Could you check a few things on this model? Use its own coordinates, in mm. Give positions to 0.01 mm unless a question says otherwise; leave off trailing zeros. Order: outer loops, then holes, each group sorted by start corner. A loop starts at its lowest first (then second) coordinate and runs counter-clockwise, first axis right, second up. Notation, with made-up numbers: M 35,13 L 65,13 A14 ccw 65,34 Z; hole C -1,86.5 d5. An arc over 180 degrees is marked long. Return JSON: item names as keys, results as strings. Group by question number.
```python
from build123d import *

# Parameters (mm, degrees)
F1_DEPTH = 5.08


# Not quite as in the source:
# - a feature names something its author has since deleted; it is built from what else it names


with BuildPart() as f1:
    # F0 (on Top) → F1 (new body)
    with BuildSketch(Plane.XY):
        with BuildLine():
            ThreePointArc((7.5830097901, 0.7499083436), (7.6107468293, 0.3754100423), (7.62, 0))
            ThreePointArc((7.62, 0), (0.4990141385, -7.6036428697), (-7.5546417033, -0.9958859045))
            ThreePointArc((-7.5546417033, -0.9958859045), (-6.3173271202, -6.8123022238), (-3.6964522326, -12.1501539452))
            ThreePointArc((-3.6964522326, -12.1501539452), (7.5612517696, -10.2037969245), (12.7, 0))
            ThreePointArc((12.7, 0), (12.5868786701, 1.6912969415), (12.249529867, 3.3524644721))
            ThreePointArc((12.249529867, 3.3524644721), (9.1791212991, 8.776886246), (3.897633179, 12.0871194088))
            ThreePointArc((3.897633179, 12.0871194088), (6.451051693, 6.6495502812), (7.5830097901, 0.7499083436))
        make_face()
        with BuildLine():
            ThreePointArc((-36.917633179, 12.0871194088), (-16.51, 23.3293611901), (3.897633179, 12.0871194088))
            ThreePointArc((3.897633179, 12.0871194088), (9.1791212991, 8.776886246), (12.249529867, 3.3524644721))
            ThreePointArc((12.249529867, 3.3524644721), (-18.3173290135, 29.0331939814), (-45.72, 0))
            ThreePointArc((-45.72, 0), (-43.286205272, 7.4762978347), (-36.917633179, 12.0871194088))
        make_face()
        with BuildLine():
            ThreePointArc((-20.32, 0), (-25.5437021653, 10.266205272), (-36.917633179, 12.0871194088))
            ThreePointArc((-36.917633179, 12.0871194088), (-43.286205272, 7.4762978347), (-45.72, 0))
            ThreePointArc((-45.72, 0), (-33.02, -12.7), (-20.32, 0))
        make_face()
        with BuildLine():
            ThreePointArc((-40.64, 0), (-40.6307468293, 0.3754100423), (-40.6030097901, 0.7499083436))
            ThreePointArc((-40.6030097901, 0.7499083436), (-32.6445899577, 7.6107468293), (-25.4, 0))
            ThreePointArc((-25.4, 0), (-33.02, -7.62), (-40.64, 0))
        make_face(mode=Mode.SUBTRACT)
        with BuildLine():
            ThreePointArc((36.7164522326, -12.1501539452), (16.51, -23.0707915841), (-3.6964522326, -12.1501539452))
            ThreePointArc((-3.6964522326, -12.1501539452), (-9.1059552655, -8.8527723739), (-12.249529867, -3.3524644721))
            ThreePointArc((-12.249529867, -3.3524644721), (18.3173290135, -29.0331939814), (45.72, 0))
            ThreePointArc((45.72, 0), (43.2237969245, -7.5612517696), (36.7164522326, -12.1501539452))
        make_face()
        with BuildLine():
            ThreePointArc((45.72, 0), (22.8162030755, 7.5612517696), (36.7164522326, -12.1501539452))
            ThreePointArc((36.7164522326, -12.1501539452), (43.2237969245, -7.5612517696), (45.72, 0))
        make_face()
        with BuildLine():
            ThreePointArc((40.64, 0), (40.6236428697, -0.4990141385), (40.5746417033, -0.9958859045))
            ThreePointArc((40.5746417033, -0.9958859045), (25.4163571303, 0.4990141385), (40.64, 0))
        make_face(mode=Mode.SUBTRACT)
        with BuildLine():
            ThreePointArc((-7.62, 0), (-0.3754100423, 7.6107468293), (7.5830097901, 0.7499083436))
            ThreePointArc((7.5830097901, 0.7499083436), (6.451051693, 6.6495502812), (3.897633179, 12.0871194088))
            ThreePointArc((3.897633179, 12.0871194088), (-8.776886246, 9.1791212991), (-12.249529867, -3.3524644721))
            ThreePointArc((-12.249529867, -3.3524644721), (-9.1059552655, -8.8527723739), (-3.6964522326, -12.1501539452))
            ThreePointArc((-3.6964522326, -12.1501539452), (-6.3173271202, -6.8123022238), (-7.5546417033, -0.9958859045))
            ThreePointArc((-7.5546417033, -0.9958859045), (-7.6036428697, -0.4990141385), (-7.62, 0))
        make_face()
    extrude(amount=F1_DEPTH)


solid = f1.part
```
1. Imagine slicing it at D-D, the plane x = -11. Please give me the cut outline in (y, z), plus the area to 3 significant figures.
2. For pin 1 (2 mm diameter, centred on x = -23, z = 4, fed in from -Y); pin 2 (1.5 mm diameter, centred on x = 34.5, z = 3, fed in from +Y); pin 3 (1.5 mm diameter, centred on x = 35.5, z = 1.5, fed in from +Y), each with a flat end and sliding along its axis, tell me the tip position at first contact or that it passes through.
3. Imagine slicing it at B-B, the plane x = 0. Please give me the cut outline in (y, z), plus the area to 3 significant figures.
4. I need wall thicknesses on L1, parallel to Y at x = 33.02, z = 3; L2, parallel to X at y = 1, z = 1.5; L3, parallel to X at y = -3, z = 1.3. Which ranges of each line are inside material? Lowest first, please. Write a range as from..to.
5. Imagine slicing it at A-A, the plane z = 1.3. Please give me the cut outline in (x, y), plus the area to 3 significant figures.
6. Imagine slicing it at C-C, the plane y = -21. Please give me the cut outline in (x, z).
7. If we mould it in two halves opening along Y, with no side actions, what happens to faces 1 (the cylindrical face through (-8.64, 9.31, 2.5)), 2 (the flat face through (-7, -4, 5.08)), 3 (the cylindrical face through (-17.702, 29.062, 2.504))? For each: pulls with the +Y half, pulls with the -Y half, needs draft (parallel to the pull), parting line crosses it, or undercut.
Values:
{
 "1": {"outline": "M -9.05,0 L 6.35,0 L 6.35,5.08 L -9.05,5.08 Z; M 22.69,0 L 28.53,0 L 28.53,5.08 L 22.69,5.08 Z", "area": "108 mm²"},
 "2": {"pin 1": "stops at y = -8.94", "pin 2": "stops at y = 12.68", "pin 3": "stops at y = 12.58"},
 "3": {"outline": "M -23.85,0 L -16.55,0 L -16.55,5.08 L -23.85,5.08 Z; M -12.7,0 L -7.62,0 L -7.62,5.08 L -12.7,5.08 Z; M 7.62,0 L 12.7,0 L 12.7,5.08 L 7.62,5.08 Z; M 16.8,0 L 23.85,0 L 23.85,5.08 L 16.8,5.08 Z", "area": "125 mm²"},
 "4": {"L1": "y = -24.03..-16.55, -12.7..-7.62, 7.62..12.7", "L2": "x = -45.7..-40.57, -25.47..-20.36, -12.66..-7.55, 7.55..12.66, 20.36..25.47, 40.57..45.68", "L3": "x = -45.36..-40.02, -26.02..-20.68, -12.34..-7, 7..12.34, 20.68..26.02, 40.02..45.56"},
 "5": {"outline": "M -45.72,0 A12.7 ccw long -36.92,12.09 A24.14 cw 3.9,12.09 A12.7 ccw -12.25,-3.35 A29.08 ccw 45.72,0 A12.7 ccw long 36.72,-12.15 A24.15 cw -3.7,-12.15 A12.7 ccw 12.25,3.35 A29.08 ccw Z; hole C -33.02,0 d15.24; hole C 0,0 d15.24; hole C 33.02,0 d15.24", "area": "1,700 mm²"},
 "6": {"outline": "M -3.48,0 L 6.72,0 L 6.72,5.08 L -3.48,5.08 Z; M 26.3,0 L 36.76,0 L 36.76,5.08 L 26.3,5.08 Z"},
 "7": {"face 1": "undercut", "face 2": "needs draft", "face 3": "pulls with the +Y half"}
}
